```python
from build123d import *

# Parameters (mm, degrees)
F1_DEPTH = 53


# Not quite as in the source:
# - a feature names something its author has since deleted; it is built from what else it names


with BuildPart() as f1:
    # F0 (on Front) → F1 (new body)
    with BuildSketch(Plane.XZ):
        Polygon((-30.7423530247, 26.6767482577), (-5.6632759116, 0.7168226163), (0.6696432283, 7.4890868759), (-21.1426665217, 29.8010575561), align=None)
        Polygon((7.143901395, 0.8665209922), (29.2684723572, 24.5259800626), (22.5106922376, 30.8453547093), (0.6696432283, 7.4890868759), align=None)
        Polygon((0.7734024336, -5.9459301822), (26.1681957986, -32.2326609282), (31.7237185496, -24.2763531905), (7.143901395, 0.8665209922), align=None)
        Polygon((-5.6632759116, 0.7168226163), (0.7734024336, -5.9459301822), (7.143901395, 0.8665209922), (0.6696432283, 7.4890868759), align=None)
        Polygon((-29.4360663926, -24.7052009039), (-22.678286273, -31.0245755505), (0.7734024336, -5.9459301822), (-5.6632759116, 0.7168226163), align=None)
    extrude(amount=-F1_DEPTH)


solid = f1.part
```
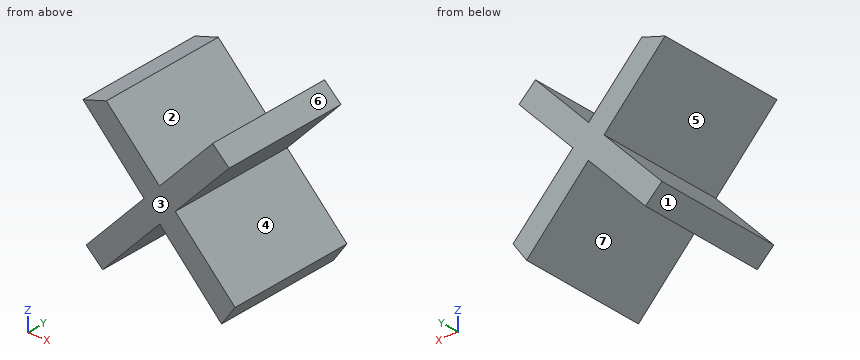
Input: part model. Units: mm. Frame: model coordinates. Face numbers are marked on the shaded views. A direction names the side the tool comes from. Coordinates: 2 decimals unless noted, no trailing zeros. Loops run counter-clockwise (first coordinate to the right, second up) from the corner with the lowest first, then second, coordinate; pieces in that order, holes last. Notation, with made-up numbers: (73.25, 55) -> (119.25, 55) arc R5 cw to (119.25, 60) -> close; hole circle Ø7 at (83.25, 3.5). An arc over 180 degrees is marked (long way). Use a Markdown table: item, result.
1) Cut plane D-D (x = -4). Return the cut outline in (y, z), then the cut area to 3 significant figures.
Results found:
| item | result |
|---|---|
| outline | (0, -11.05) -> (53, -11.05) -> (53, 12.27) -> (0, 12.27) -> close |
| area | 1,240 mm2 |
2) Contact query for flat-ended pins moving along their axis: pin 1 (8 mm diameter, centred on y = 31, z = 22.5, fed in from +X); pin 2 (10 mm diameter, centred on y = 44.5, z = 0.5, fed in from +X); pin 3 (12 mm diameter, centred on y = 46, z = -22, fed in from +X). Output: stop coordinate, or through.
Results found:
| item | result |
|---|---|
| pin 1 | stops at x = 29.27 |
| pin 2 | stops at x = 12.39 |
| pin 3 | stops at x = 31.72 |
3) Material intervals for line 1 along Z through (x, y) = (-17, 46.5); line 2 along X through (y, z) = (47, -29); line 3 along X through (y, z) = (28, 17), sorted ascending. Write a range as from..to.
Results found:
| item | result |
|---|---|
| line 1 | z = -24.95..-11.41, 12.45..25.56 |
| line 2 | x = -24.84..-20.79, 23.05..28.43 |
| line 3 | x = -21.39..-8.63, 9.56..22.23 |
4) Cut plane A-A (z = -10). Return the cut outline in (x, y).
Results found:
| item | result |
|---|---|
| outline | (-15.68, 0) -> (-3.02, 0) -> (-3.02, 53) -> (-15.68, 53) -> close; (4.69, 0) -> (17.77, 0) -> (17.77, 53) -> (4.69, 53) -> close |
5) Cut plane C-C (y = 22). Return the cut outline in (x, z).
Results found:
| item | result |
|---|---|
| outline | (-30.74, 26.68) -> (-5.66, 0.72) -> (-29.44, -24.71) -> (-22.68, -31.02) -> (0.77, -5.95) -> (26.17, -32.23) -> (31.72, -24.28) -> (7.14, 0.87) -> (29.27, 24.53) -> (22.51, 30.85) -> (0.67, 7.49) -> (-21.14, 29.8) -> close |
6) Cut plane B-B (x = 24). Return the cut outline in (y, z).
Results found:
| item | result |
|---|---|
| outline | (0, -29.99) -> (53, -29.99) -> (53, -16.38) -> (0, -16.38) -> close; (0, 18.89) -> (53, 18.89) -> (53, 29.45) -> (0, 29.45) -> close |
7) Pull-direction query (Z, two-part tool) for the marked faces 1, 2, 3 and 4; classes: released by +Z, released by -Z, zero draft, split by the parting line, or undercut.
Results found:
| item | result |
|---|---|
| face 1 | released by -Z |
| face 2 | released by +Z |
| face 3 | zero draft |
| face 4 | undercut |
8) Access query for the marked faces 5, 6 and 7. Directions: +Z, -Z, +X, -X, +Y, -Y. A direction counts if a zero-diameter tool reaches every point of the face in a straight line with its end or side. Return the directions, or none.
Results found:
| item | result |
|---|---|
| face 5 | -X, +Y, -Y |
| face 6 | +Z, +X, +Y, -Y |
| face 7 | -Z, +Y, -Y |
